from build123d import *

# Parameters (mm, degrees)
ESBO_O1_R                = 17.5
RESSALTO_EXTRUS_O1_DEPTH = 5
ESBO_O2_R                = 10
RESSALTO_EXTRUS_O2_DEPTH = 10
ESBO_O3_R                = 7.5
CORTE_EXTRUS_O1_DEPTH    = 16
ESBO_O4_R                = 1.5
CORTE_EXTRUS_O2_DEPTH    = 10
ESBO_O5_R                = 1.5
CORTE_EXTRUS_O3_DEPTH    = 10
ESBO_O6_R                = 1.5
CORTE_EXTRUS_O4_DEPTH    = 10


with BuildPart() as part:
    # Esboço1 → Ressalto-extrusão1 (new body)
    with BuildSketch(Plane(origin=(0, 0, 0), x_dir=(1, 0, 0), z_dir=(0, 1, 0))):
        Circle(ESBO_O1_R)
    extrude(amount=RESSALTO_EXTRUS_O1_DEPTH)

    # Esboço2 → Ressalto-extrusão2 (add)
    with BuildSketch(Plane(origin=(0, 5, 0), x_dir=(1, 0, 0), z_dir=(0, 1, 0))):
        Circle(ESBO_O2_R)
    extrude(amount=RESSALTO_EXTRUS_O2_DEPTH)

    # Esboço3 → Corte-extrusão1 (cut, through all)
    with BuildSketch(Plane(origin=(0, 15, 0), x_dir=(1, 0, 0), z_dir=(0, 1, 0))):
        Circle(ESBO_O3_R)
    extrude(amount=-CORTE_EXTRUS_O1_DEPTH, mode=Mode.SUBTRACT)

    # Esboço4 → Corte-extrusão2 (cut)
    with BuildSketch(Plane(origin=(0, 5, 0), x_dir=(1, 0, 0), z_dir=(0, 1, 0))):
        with Locations((0, 13.75)):
            Circle(ESBO_O4_R)
        with Locations((0, -13.75)):
            Circle(ESBO_O4_R)
    extrude(amount=-CORTE_EXTRUS_O2_DEPTH, mode=Mode.SUBTRACT)

    # Esboço5 → Corte-extrusão3 (cut)
    with BuildSketch(Plane.XY):
        with Locations((0, 10)):
            Circle(ESBO_O5_R)
    extrude(amount=-CORTE_EXTRUS_O3_DEPTH, mode=Mode.SUBTRACT)

    # Esboço6 → Corte-extrusão4 (cut)
    with BuildSketch(Plane(origin=(0, 0, 0), x_dir=(0, 0, -1), z_dir=(1, 0, 0))):
        with Locations((0, 10)):
            Circle(ESBO_O6_R)
    extrude(amount=-CORTE_EXTRUS_O4_DEPTH, mode=Mode.SUBTRACT)


solid = part.part
Could you check a few things on this model? Use its own coordinates, in mm. A direction names the side the tool comes from. Give positions to 0.01 mm unless a question says otherwise; leave off trailing zeros. Order: outer loops, then holes, each group sorted by start corner. A loop starts at its lowest first (then second) coordinate and runs counter-clockwise, first axis right, second up. Notation, with made-up numbers: (-39.75, 89) -> (-22.75, 89) arc R12 ccw to (-22.75, 104) -> close; hole circle Ø2 at (-24, 88). An arc over 180 degrees is marked (long way). Answer in a Markdown table with one row per item. Add a question column.
Item 1: Imagine slicing it at A-A (x = 0). List the corners of the cut face in (y, z) for me, and give its area (4 significant figures).
Item 2: Please list where these lines run through material, in increasing order: probe 1 along Y at (x, z) = (0, -9.3); probe 2 along Y at (x, z) = (3, -14); probe 3 along X at (y, z) = (2.2, -13.75).
Item 3: For faces 1 (the cylindrical face through (9.237, 9.93, 3.83)), 2 (the cylindrical face through (-8.656, 9.425, -1.386)), 3 (the cylindrical face through (-0.325, 2.535, 15.214)), which set-ups out of +Z, -Z, +X, -X, +Y, -Y let a thin tool reach every point of the face, with its end or its side?
Item 4: I'm going to push flat-ended pins straight in: P1, Ø1.8, axis at y = 10, z = 0, coming from the -X side; P2, Ø3, axis at x = -5.5, y = 13.5, coming from the -Z side; P3, Ø10, axis at x = -5, z = -1.5, coming from the +Y side; P4, Ø5, axis at y = 12, z = 4, coming from the -X side. Where does each tip first touch, or does it pass through?
Item 5: We'd pull the mould along Y, two halves only. Please class faces 4 (the cylindrical face through (-13.887, 2.465, 10.648)), 5 (the cylindrical face through (1.386, 9.425, -8.654)), 6 (the flat face through (8, 5, 8)): pulls with the +Y half, pulls with the -Y half, needs draft (parallel to the pull), parting line crosses it, or undercut.
Item 6: Imagine slicing it at C-C (y = 10). List the corners of the cut face in (x, z) for me.
Item 7: Imagine slicing it at B-B (z = -3). List the corners of the cut face in (x, y) for me, and give its area (3 significant figures).
Item 8: Imagine slicing it at D-D (x = -6). List the corners of the cut face in (y, z) for me.
Result:
| question | item | result |
|---|---|---|
| 1 | outline | (0, -17.5) -> (5, -17.5) -> (5, -15.25) -> (0, -15.25) -> close; (0, -12.25) -> (5, -12.25) -> (5, -10) -> (8.5, -10) -> (8.5, -7.5) -> (0, -7.5) -> close; (0, 7.5) -> (15, 7.5) -> (15, 10) -> (5, 10) -> (5, 12.25) -> (0, 12.25) -> close; (0, 15.25) -> (5, 15.25) -> (5, 17.5) -> (0, 17.5) -> close; (11.5, -10) -> (15, -10) -> (15, -7.5) -> (11.5, -7.5) -> close |
| 1 | area | 112.5 mm2 |
| 2 | probe 1 | 0 to 8.5, 11.5 to 15 |
| 2 | probe 2 | 0 to 5 |
| 2 | probe 3 | -10.83 to -1.5, 1.5 to 10.83 |
| 3 | face 1 | +Y |
| 3 | face 2 | -X |
| 3 | face 3 | +Y, -Y |
| 4 | P1 | x = 7.45 |
| 4 | P2 | z = -9.17 |
| 4 | P3 | y = 15 |
| 4 | P4 | x = -9.89 |
| 5 | face 4 | needs draft |
| 5 | face 5 | undercut |
| 5 | face 6 | pulls with the +Y half |
| 6 | outline | (-9.89, -1.5) arc R10 ccw to (-1.5, -9.89) -> (-1.5, -7.35) arc R7.5 cw to (-7.35, -1.5) -> close; (-9.89, 1.5) -> (-7.35, 1.5) arc R7.5 cw (long way) to (1.5, -7.35) -> (1.5, -9.89) arc R10 ccw (long way) to start |
| 7 | outline | (-17.24, 0) -> (-6.87, 0) -> (-6.87, 15) -> (-9.54, 15) -> (-9.54, 5) -> (-17.24, 5) -> close; (6.87, 0) -> (17.24, 0) -> (17.24, 5) -> (9.54, 5) -> (9.54, 15) -> (6.87, 15) -> close |
| 7 | area | 157 mm2 |
| 8 | outline | (0, -16.44) -> (5, -16.44) -> (5, -8) -> (15, -8) -> (15, -4.5) -> (0, -4.5) -> close; (0, 4.5) -> (15, 4.5) -> (15, 8) -> (5, 8) -> (5, 16.44) -> (0, 16.44) -> close |
